from build123d import *

# Parameters (mm, degrees)
F0_R     = 9.85
F1_DEPTH = 34
F3_DEPTH = 27
F5_DEPTH = 3


with BuildPart() as f1:
    # F0 (on Top) → F1 (new body)
    with BuildSketch(Plane.XY):
        Circle(F0_R)
    extrude(amount=F1_DEPTH)

    # F2 (on face) → F3 (cut)
    with BuildSketch(Plane.XY.offset(34)):
        with BuildLine():
            Line((-9.85, 0), (9.85, 0))
            ThreePointArc((9.85, 0), (0, 9.85), (-9.85, 0))
        make_face()
    extrude(amount=-F3_DEPTH, mode=Mode.SUBTRACT)

    # F4 (on face) → F5 (cut)
    with BuildSketch(Plane.XY.offset(7)):
        with BuildLine():
            ThreePointArc((-9.00125, 4), (-9.635476, 2.044528), (-9.85, 0))
            Line((-9.85, 0), (9.85, 0))
            ThreePointArc((9.85, 0), (9.635476, 2.044528), (9.00125, 4))
            Line((9.00125, 4), (4.553003, 4))
            Line((4.553003, 4), (4.553003, 5))
            Line((4.553003, 5), (-4.553003, 5))
            Line((-4.553003, 5), (-4.553003, 4))
            Line((-4.553003, 4), (-9.00125, 4))
        make_face()
    extrude(amount=-F5_DEPTH, mode=Mode.SUBTRACT)


solid = f1.part
Can you work these out from the model? Positions are in its coordinate system, mm. A direction names the side the tool comes from. Give positions to 0.01 mm unless a question says otherwise; leave off trailing zeros. Write each loop counter-clockwise with the first axis right and the second up, starting at its lowest first coordinate (ties: lowest second). Pieces come first, ordered by that corner, then holes. Notation, with made-up numbers: (-31, 45.5) -> (-8, 45.5) arc R18 cw to (-8, 60.5) -> close; hole circle Ø10 at (74.25, 50). An arc over 180 degrees is marked (long way). Answer as a JSON object with one key per item and string values. Group by question number.
Item 1: Suppose I cut it at C-C (y = -2.5). Please give me the cut outline in (x, z).
Item 2: We'd pull the mould along Y, two halves only. Please class faces 5 (the face through (0, 0, 0)), 6 (the face through (7, 4, 6)), 7 (the face through (-2.135, -9.616, 12.984)): +Y half, -Y half, draft (parallel to the pull), parting line (faces both ways), or undercut.
Item 3: Suppose I cut it at B-B (z = 9.5). Please give me the cut outline in (x, y), plus the area to 3 significant figures.
Item 4: For faces 1 (the face through (0, -4, 34)), 2 (the face through (4.553, 4.5, 5.5)), 3 (the face through (0, 7, 7)), 4 (the face through (-7, 4, 6)), which set-ups out of +Z, -Z, +X, -X, +Y, -Y let a thin tool reach every point of the face, with its end or its side?
Item 5: Please list where these lines run through material, in increasing order: line 1 (Z direction, x = -3.5, y = 3.25); line 2 (Y direction, x = 0, z = 10); line 3 (Z direction, x = 2.75, y = 8.25). Write a range as [from, to].
Item 6: I'm going to push flat-ended pins straight in: P1, Ø1.5, axis at x = 5.5, z = 21, coming from the +Y side; P2, Ø1.8, axis at x = 1, y = 7.5, coming from the +Z side; P3, Ø1.5, axis at x = 7, z = 5.5, coming from the -Y side; P4, Ø6, axis at x = 0.5, y = 1, coming from the -Z side. Where does each tip first touch, or does it pass through?
Item 7: Suppose I cut it at A-A (x = 0). Please give me the cut outline in (y, z), plus the area to 3 significant figures.
Item 8: Suppose I cut it at D-D (x = -5). Please give me the cut outline in (y, z).
Findings:
{
 "1": {"outline": "(-9.53, 0) -> (9.53, 0) -> (9.53, 34) -> (-9.53, 34) -> close"},
 "2": {"face 5": "draft", "face 6": "undercut", "face 7": "parting line"},
 "3": {"outline": "(-9.85, 0) arc R9.85 ccw to (9.85, 0) -> close", "area": "152 mm²"},
 "4": {"face 1": "+Z, +X, -X, +Y, -Y", "face 2": "+Z", "face 3": "+Z, +X, -X, +Y", "face 4": "+Z, +X, -X"},
 "5": {"line 1": "z = [0, 4]", "line 2": "y = [-9.85, 0]", "line 3": "z = [0, 7]"},
 "6": {"P1": "stops at y = 0", "P2": "stops at z = 7", "P3": "stops at y = -7.61", "P4": "stops at z = 0"},
 "7": {"outline": "(-9.85, 0) -> (9.85, 0) -> (9.85, 7) -> (5, 7) -> (5, 4) -> (0, 4) -> (0, 34) -> (-9.85, 34) -> close", "area": "389 mm²"},
 "8": {"outline": "(-8.49, 0) -> (8.49, 0) -> (8.49, 7) -> (4, 7) -> (4, 4) -> (0, 4) -> (0, 34) -> (-8.49, 34) -> close"}
}
